from build123d import *

# Parameters (mm, degrees)
F0_W      = 28
F0_H      = 200
F1_DEPTH  = 54.356
F3_W      = 27.69987
F3_H      = 91.44
F4_DEPTH  = 33
F4_FACE_W = 33
F4_FACE_H = 91.44
F5_DEPTH  = 25.4
F6_R      = 2.778125
F7_DEPTH  = 12.7
F8_W      = 54.356
F8_H      = 29.860789
F9_DEPTH  = 38.1
F10_W     = 54.356
F10_H     = 29.860789
F11_DEPTH = 38.1


with BuildPart() as f1:
    # F0 (on Front) → F1 (new body)
    with BuildSketch(Plane.XZ):
        with Locations((-41.935609, 69.564922)):
            Rectangle(F0_W, F0_H)
    extrude(amount=F1_DEPTH)

    # F3 (on face) → F4 (cut)
    with BuildSketch(Plane.XZ.offset(54.356)):
        with Locations((-41.785544, 75.0065)):
            Rectangle(F3_W, F3_H)
    extrude(amount=-F4_DEPTH, mode=Mode.SUBTRACT)

    # F4_face (on face) → F5 (cut)
    with BuildSketch(Plane(origin=(-55.635479, -37.856, 75.0065), x_dir=(0, 1, 0), z_dir=(1, 0, 0))):
        Rectangle(F4_FACE_W, F4_FACE_H)
    extrude(amount=-F5_DEPTH, mode=Mode.SUBTRACT)

    # F6 (on face) → F7 (cut)
    with BuildSketch(Plane.XZ.offset(54.356)):
        with Locations((-41.935609, 145)):
            Circle(F6_R)
        with Locations((-41.935609, 5)):
            Circle(F6_R)
    extrude(amount=-F7_DEPTH, mode=Mode.SUBTRACT)

    # F8 (on face) → F9 (join)
    with BuildSketch(Plane.YZ.offset(-27.935609)):
        with Locations((-27.178, -15.504683)):
            Rectangle(F8_W, F8_H)
    extrude(amount=F9_DEPTH)

    # F10 (on face) → F11 (join)
    with BuildSketch(Plane(origin=(-55.935609, 0, 0), x_dir=(0, -1, 0), z_dir=(-1, 0, 0))):
        with Locations((27.178, -15.504683)):
            Rectangle(F10_W, F10_H)
    extrude(amount=F11_DEPTH)


solid = f1.part
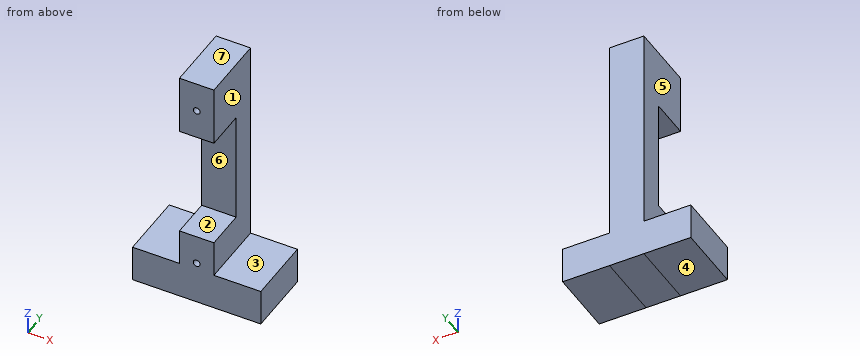
Read the model definition and answer for the solid it produces. Units are mm, in the model's axes. Face numbers are marked on the shaded views. A direction names the side the tool comes from. Round coordinates to 2 decimals unless told otherwise and drop trailing zeros. Order: outer loops, then holes, each group sorted by start corner. A loop starts at its lowest first (then second) coordinate and runs counter-clockwise, first axis right, second up.
1) Flat-ended cylindrical pins translate along their axes: pin 1 (19 mm diameter, centred on x = -83, y = -30.5, fed in from +Z); pin 2 (7 mm diameter, centred on x = -41.94, z = 5, fed in from -Y); pin 3 (22.5 mm diameter, centred on x = -35, z = 63, fed in from -Y); pin 4 (12 mm diameter, centred on y = -34, z = 26, fed in from -X). Find the tip coordinate at first contact, or state that the pin passes through.
2) The part is cut by section C-C on x = -32.5. Write down the section's boundary in (y, z).
3) The part is cut by section B-B on z = 5. Write down the section's boundary in (x, y).
4) The mould has two halves that part along Z. Classify the marked faces 1, 2, 3 and 4: released by +Z, released by -Z, zero draft, split by the parting line, or undercut.
5) For the marked faces 5, 6 and 7, determine the directions among +Z, -Z, +X, -X, +Y, -Y from which every point of the face is accessible in a straight line to the end or side of a thin tool.
6) The part is cut by section D-D on y = -11. Write down the section's boundary in (x, z).
7) Straight lines are drawn through the part: L1, parallel to Z at x = -45, y = -25.5; L2, parallel to Z at x = -87.5, y = -12; L3, parallel to X at y = -4, z = 85. For each, find the intervals that lie inside material, in ascending order.
8) The part is cut by section A-A on y = -45.5. Write down the section's boundary in (x, z).
Resolved:
1. pin 1: stops at z = -0.57
1. pin 2: stops at y = -54.36
1. pin 3: stops at y = -21.36
1. pin 4: stops at x = -55.94
2. outline: (-54.36, -30.44) - (0, -30.44) - (0, 169.56) - (-54.36, 169.56) - (-54.36, 120.73) - (-21.36, 120.73) - (-21.36, 29.29) - (-54.36, 29.29) - close
3. outline: (-55.94, -54.36) - (-44.71, -54.36) - (-44.71, -41.66) - (-39.16, -41.66) - (-39.16, -54.36) - (-27.94, -54.36) - (-27.94, 0) - (-55.94, 0) - close
4. face 1: zero draft
4. face 2: undercut
4. face 3: released by +Z
4. face 4: released by -Z
5. face 5: +Z, -X, +Y, -Y
5. face 6: +X, -X, -Y
5. face 7: +Z, +X, -X, +Y, -Y
6. outline: (-94.04, -30.44) - (10.16, -30.44) - (10.16, -0.57) - (-27.94, -0.57) - (-27.94, 169.56) - (-55.94, 169.56) - (-55.94, -0.57) - (-94.04, -0.57) - close
7. L1: z = -30.44 to 29.29, 120.73 to 169.56
7. L2: z = -30.44 to -0.57
7. L3: x = -55.94 to -27.94
8. outline: (-94.04, -30.44) - (10.16, -30.44) - (10.16, -0.57) - (-27.94, -0.57) - (-27.94, 29.29) - (-55.94, 29.29) - (-55.94, -0.57) - (-94.04, -0.57) - close; (-55.94, 120.73) - (-27.94, 120.73) - (-27.94, 169.56) - (-55.94, 169.56) - close; hole circle Ø5.56 at (-41.94, 5); hole circle Ø5.56 at (-41.94, 145)
